Check sheet for the modelled part. Datum: model origin and axes. Units: mm. Coordinates: 2 decimals unless noted, no trailing zeros. Order: outer loops, then holes, each group sorted by start corner. A loop starts at its lowest first (then second) coordinate and runs counter-clockwise, first axis right, second up.
1. Draft check along Z on faces 1 (the cylindrical face through (20.504, 4.93, 36.038)), 2 (the flat face through (80, 5, 0)), 3 (the cylindrical face through (-77.15, 5.07, 41.99)). Enter one of: released by +Z, released by -Z, zero draft, split by the parting line, or undercut.
2. Cross-section at A-A (y = 4.75). Count the separate pieces of the cut face and the enclosed holes in it, then the cut area to 3 significant figures.
3. Gauge pin test, flat end, axial feed: pin 1 Ø1.5 at (x, z) = (61, 30) entering from -Y. Record the tip position at first contact, or that the pin passes through.
4. Thickness scan on line 1 (Z direction, x = 44, y = 5.5); line 2 (Z direction, x = -20.5, y = 4.5); line 3 (X direction, y = 1.5, z = -37.5). Record the ranges inside material, lowest first.
5. Cross-section at B-B (x = 45). Enter the section's corners in (y, z), then the cut area to 3 significant figures.
```python
from build123d import *

# Parameters (mm, degrees)
SKETCH1_W           = 160
SKETCH1_H           = 90
SKETCH1_R           = 2.25
BOSS_EXTRUDE1_DEPTH = 10
FILLET1_R           = 10


with BuildPart() as part:
    # Sketch1 → Boss-Extrude1 (new body)
    with BuildSketch(Plane(origin=(0, 0, 0), x_dir=(1, 0, 0), z_dir=(0, 1, 0))):
        Rectangle(SKETCH1_W, SKETCH1_H)
        with Locations(Location((-67.5, 35, 0), (0, 0, 270))):
            Circle(SKETCH1_R, mode=Mode.SUBTRACT)
        with Locations(Location((-22.5, 35, 0), (0, 0, 270))):
            Circle(SKETCH1_R, mode=Mode.SUBTRACT)
        with Locations(Location((22.5, 35, 0), (0, 0, 270))):
            Circle(SKETCH1_R, mode=Mode.SUBTRACT)
        with Locations(Location((67.5, 35, 0), (0, 0, 270))):
            Circle(SKETCH1_R, mode=Mode.SUBTRACT)
        with Locations(Location((67.5, -35, 0), (0, 0, 270))):
            Circle(SKETCH1_R, mode=Mode.SUBTRACT)
        with Locations(Location((22.5, -35, 0), (0, 0, 270))):
            Circle(SKETCH1_R, mode=Mode.SUBTRACT)
        with Locations(Location((-22.5, -35, 0), (0, 0, 270))):
            Circle(SKETCH1_R, mode=Mode.SUBTRACT)
        with Locations(Location((-67.5, -35, 0), (0, 0, 270))):
            Circle(SKETCH1_R, mode=Mode.SUBTRACT)
        with Locations(Location((-45, 35, 0), (0, 0, 270))):
            Circle(SKETCH1_R, mode=Mode.SUBTRACT)
        with Locations(Location((45, 35, 0), (0, 0, 270))):
            Circle(SKETCH1_R, mode=Mode.SUBTRACT)
        with Locations(Location((0, 35, 0), (0, 0, 270))):
            Circle(SKETCH1_R, mode=Mode.SUBTRACT)
        with Locations(Location((-45, -35, 0), (0, 0, 270))):
            Circle(SKETCH1_R, mode=Mode.SUBTRACT)
        with Locations(Location((0, -35, 0), (0, 0, 270))):
            Circle(SKETCH1_R, mode=Mode.SUBTRACT)
        with Locations(Location((45, -35, 0), (0, 0, 270))):
            Circle(SKETCH1_R, mode=Mode.SUBTRACT)
    extrude(amount=BOSS_EXTRUDE1_DEPTH)

    # Fillet1
    fillet1_edges = [part.edges().sort_by_distance(p)[0] for p in [
        (-80, 5, -45),
        (80, 5, -45),
        (80, 5, 45),
        (-80, 5, 45),
    ]]
    fillet(fillet1_edges, radius=FILLET1_R)


solid = part.part
```
Data:
1. face 1: undercut
1. face 2: zero draft
1. face 3: released by +Z
2. separate pieces: 1
2. enclosed holes: 14
2. area: 14,100 mm2
3. pin 1: stops at y = 0
4. line 1: z = -45 to -37.02, -32.98 to 32.98, 37.02 to 45
4. line 2: z = -45 to -36.03, -33.97 to 33.97, 36.03 to 45
4. line 3: x = -79.68 to 79.68
5. outline: (0, -45) - (10, -45) - (10, -37.25) - (0, -37.25) - close; (0, -32.75) - (10, -32.75) - (10, 32.75) - (0, 32.75) - close; (0, 37.25) - (10, 37.25) - (10, 45) - (0, 45) - close
5. area: 810 mm2
